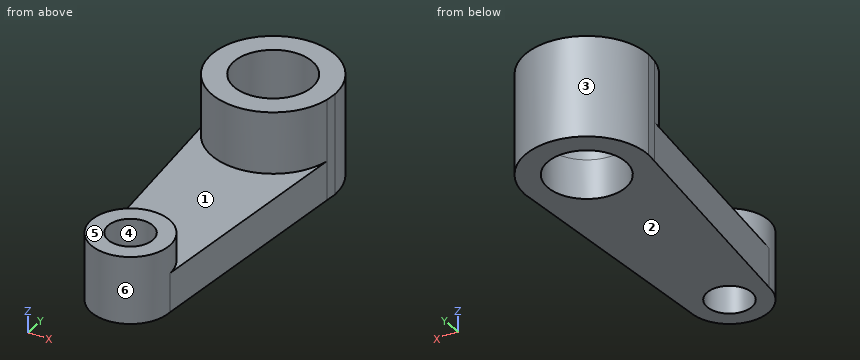
```python
from build123d import *

# Parameters (mm, degrees)
F0_R     = 22.225
F0_R_2   = 12.7
F1_DEPTH = 22.225
F2_R     = 22.225
F3_DEPTH = 34.925
F4_DEPTH = 50.8
F5_R     = 12.7
F6_DEPTH = 15.875
F7_R     = 12.7
F8_DEPTH = 38.1


# Not quite as in the source:
# - a length typed as a fraction of an inch, garbled in the dataset ("3 / 203.2 mm" for 3/8 in), is restored


with BuildPart() as f1:
    # F0 (on Top) → F1 (new body)
    with BuildSketch(Plane.XY):
        with BuildLine():
            Line((22.225, 0), (34.2971348315, 126.7574157303))
            ThreePointArc((34.2971348315, 126.7574157303), (0, 98.425), (-34.2971348315, 126.7574157303))
            Line((-34.2971348315, 126.7574157303), (-22.225, 0))
            ThreePointArc((-22.225, 0), (0, 22.225), (22.225, 0))
        make_face()
        with BuildLine():
            Line((34.2971348315, 126.7574157303), (34.925, 133.35))
            ThreePointArc((34.925, 133.35), (0, 168.275), (-34.925, 133.35))
            Line((-34.925, 133.35), (-34.2971348315, 126.7574157303))
            ThreePointArc((-34.2971348315, 126.7574157303), (0, 98.425), (34.2971348315, 126.7574157303))
        make_face()
        with Locations((0, 133.35)):
            Circle(F0_R, mode=Mode.SUBTRACT)
        with BuildLine():
            ThreePointArc((-22.225, 0), (0, -22.225), (22.225, 0))
            ThreePointArc((22.225, 0), (0, 22.225), (-22.225, 0))
        make_face()
        Circle(F0_R_2, mode=Mode.SUBTRACT)
        with Locations((0, 133.35)):
            Circle(F0_R)
        Circle(F0_R_2)
    extrude(amount=F1_DEPTH)

    # F2 (on face) → F3 (join)
    with BuildSketch(Plane.XY.offset(22.225)):
        with BuildLine():
            ThreePointArc((-34.2971348315, 126.7574157303), (0, 98.425), (34.2971348315, 126.7574157303))
            Line((34.2971348315, 126.7574157303), (34.925, 133.35))
            ThreePointArc((34.925, 133.35), (0, 168.275), (-34.925, 133.35))
            Line((-34.925, 133.35), (-34.2971348315, 126.7574157303))
        make_face()
        with Locations((0, 133.35)):
            Circle(F2_R, mode=Mode.SUBTRACT)
    extrude(amount=F3_DEPTH)

    # F4 (cut): a face of the model
    f4_faces = [f1.faces().sort_by_distance(p)[0] for p in [
        (0, 133.35, 22.225),
    ]]
    extrude(f4_faces, amount=-F4_DEPTH, mode=Mode.SUBTRACT)

    # F5 (on face) → F6 (join)
    with BuildSketch(Plane.XY.offset(22.225)):
        with BuildLine():
            ThreePointArc((-22.225, 0), (0, -22.225), (22.225, 0))
            ThreePointArc((22.225, 0), (0, 22.225), (-22.225, 0))
        make_face()
        Circle(F5_R, mode=Mode.SUBTRACT)
        Circle(F5_R)
    extrude(amount=F6_DEPTH)

    # F7 (on face) → F8 (cut)
    with BuildSketch(Plane.XY.offset(38.1)):
        Circle(F7_R)
    extrude(amount=-F8_DEPTH, mode=Mode.SUBTRACT)


solid = f1.part
```
Design review of the part built by this model. Coordinates are the model's own, in mm. Face numbers are marked on the shaded views. A direction names the side the tool comes from. Coordinates: 2 decimals unless noted, no trailing zeros. Order: outer loops, then holes, each group sorted by start corner. A loop starts at its lowest first (then second) coordinate and runs counter-clockwise, first axis right, second up.
1) Mouldability with a two-part tool opening along Y and no side actions: class the marked faces 1, 2 and 3 as +Y half, -Y half, draft (parallel to the pull), parting line (faces both ways), or undercut.
2) Take a section at C-C, the plane z = 7.5. Give the boundary of the cut face in (x, y) (3 decimals).
3) Clearance check with flat-ended pins moving along their axes: pin 1 (5 mm diameter, centred on x = 4.5, z = 18, fed in from +Y); pin 2 (10 mm diameter, centred on y = 102, z = 19.5, fed in from +X); pin 3 (6 mm diameter, centred on x = 0.5, y = 41.5, fed in from +Z) (3 decimals); pin 4 (15 mm diameter, centred on x = 0, y = 0, fed in from +Z). State where each tip first meets the part, or that it passes through.
4) Take a section at B-B, the plane x = 0. Give the boundary of the cut face in (y, z) (3 decimals).
5) Take a section at A-A, the plane x = -15. Give the boundary of the cut face in (y, z) (3 decimals).
6) For the marked faces 4, 5 and 6, list the 3-axis set-ups (+Z, -Z, +X, -X, +Y, -Y) from which the entire face can be reached by the end or side of a thin tool; tool diameter is ignored.
7) Wall thickness on line 1 along Y through (x, z) = (0, 12.5) (3 decimals); line 2 along Y through (x, z) = (0, 28) (3 decimals); line 3 along Y through (x, z) = (0, 46) (3 decimals): over which ranges is each line inside the solid? List them lowest first.
8) Take a section at D-D, the plane z = 50. Give the boundary of the cut face in (x, y) (3 decimals), and give its area (3 significant figures).
Returned:
1. face 1: undercut
1. face 2: draft
1. face 3: +Y half
2. outline: (-34.925, 133.35) - (-22.225, 0) arc R22.225 ccw to (22.225, 0) - (34.925, 133.35) arc R34.925 ccw to start; hole circle Ø44.45 at (0, 133.35); hole circle Ø25.4 at (0, 0)
3. pin 1: stops at y = 168.22
3. pin 2: stops at x = 32.42
3. pin 3: stops at z = 22.225
3. pin 4: passes through
4. outline: (-22.225, 0) - (-12.7, 0) - (-12.7, 38.1) - (-22.225, 38.1) - close; (12.7, 0) - (111.125, 0) - (111.125, 57.15) - (98.425, 57.15) - (98.425, 22.225) - (22.225, 22.225) - (22.225, 38.1) - (12.7, 38.1) - close; (155.575, 0) - (168.275, 0) - (168.275, 57.15) - (155.575, 57.15) - close
5. outline: (-16.4, 0) - (116.95, 0) - (116.95, 57.15) - (101.81, 57.15) - (101.81, 22.225) - (16.4, 22.225) - (16.4, 38.1) - (-16.4, 38.1) - close; (149.75, 0) - (164.89, 0) - (164.89, 57.15) - (149.75, 57.15) - close
6. face 4: +Z, -Z
6. face 5: +Z, +X, -X, -Y
6. face 6: +Z
7. line 1: y = -22.225 to -12.7, 12.7 to 111.125, 155.575 to 168.275
7. line 2: y = -22.225 to -12.7, 12.7 to 22.225, 98.425 to 111.125, 155.575 to 168.275
7. line 3: y = 98.425 to 111.125, 155.575 to 168.275
8. outline: (-34.925, 133.35) - (-34.297, 126.757) arc R34.925 ccw to (34.297, 126.757) - (34.925, 133.35) arc R34.925 ccw to start; hole circle Ø44.45 at (0, 133.35)
8. area: 2,280 mm2
